Geometry: see drawing. Coordinates: mm, zero at the bounding-box minimum. A direction names the side the tool comes from. Round coordinates to 2 decimals unless told otherwise and drop trailing zeros. Write each loop counter-clockwise with the first axis right and the second up, starting at its lowest first coordinate (ties: lowest second). Pieces come first, ordered by that corner, then holes. Notation, with made-up numbers: M 12.5,-28 L 40.5,-28 A22 ccw 40.5,3 Z; hole C 5.5,31 d5. An arc over 180 degrees is marked long. Use one line per item in the form item = value. Start each with the question number.
Item 1: Reachability of the marked faces 4, 5 and 6 from +Z, -Z, +X, -X, +Y, -Y: full face, straight path, thin tool, end or side. Return the list, or none.
Item 2: Section query B-B (y = 10). Return loops of the section in (x, z), and give its area (3 significant figures).
Item 3: Pin query (flat end, axial travel): pin 1 Ø7 at (x, y) = (10, 10) entering from +Z; pin 2 Ø4 at (x, z) = (3.5, 8) entering from -Y. Return the tip coordinate at first contact, or that it passes through.
Item 4: Pull-direction query (X, two-part tool) for the marked faces 1, 2 and 3; classes: pulls with the +X half, pulls with the -X half, needs draft (parallel to the pull), parting line crosses it, or undercut.
Item 5: Section query A-A (x = 10). Return loops of the section in (y, z).
Item 6: Section query C-C (z = 7.5). Return loops of the section in (x, y), and give its area (3 significant figures).
Item 7: Ray query, probe 1 along Y at (x, z) = (10, 2.25); probe 2 along X at (y, z) = (62, 9.25); probe 3 along Y at (x, z) = (10.5, 2.25). Return the intervals inside material, ascending.
Item 8: Section query D-D (y = 36). Return loops of the section in (x, z).
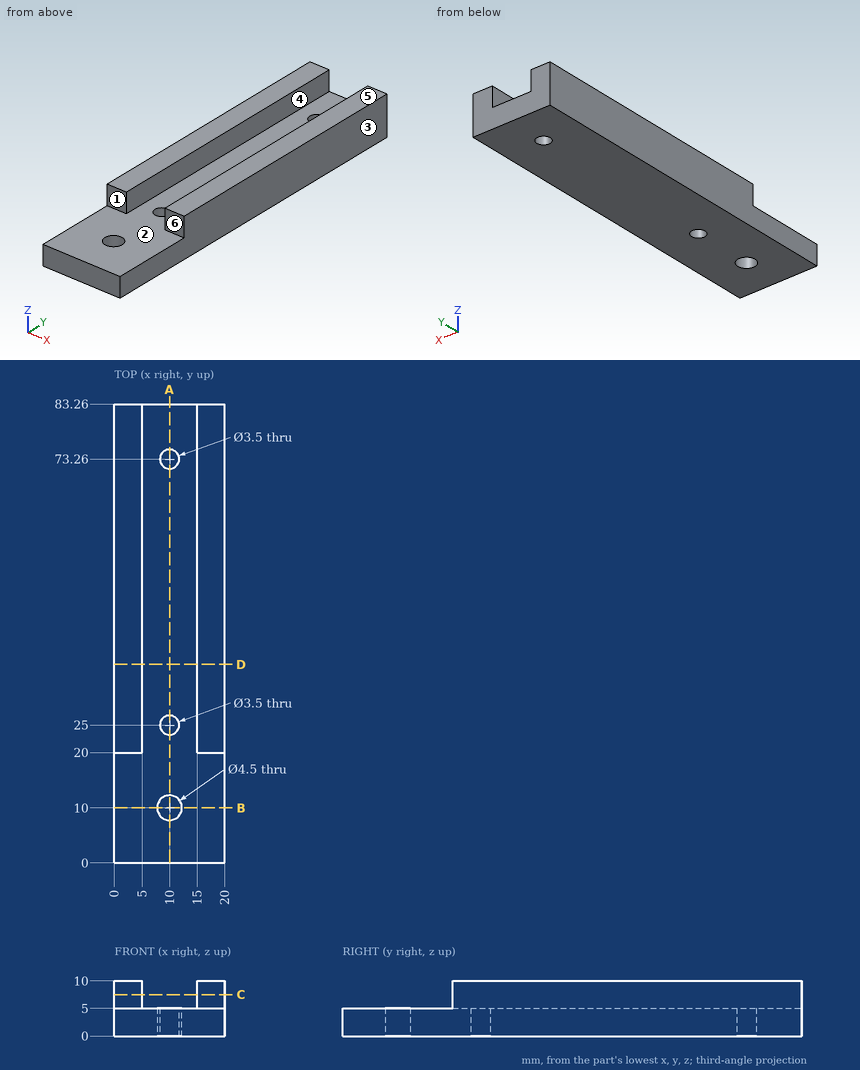
Working result:
q1.face_4 = +Z, +Y, -Y
q1.face_5 = +Z, +X, -X, +Y, -Y
q1.face_6 = +Z, +X, -X, -Y
q2.outline = M 0,0 L 7.75,0 L 7.75,5 L 0,5 Z; M 12.25,0 L 20,0 L 20,5 L 12.25,5 Z
q2.area = 77.5 mm²
q3.pin_1 = 5
q3.pin_2 = 20
q4.face_1 = needs draft
q4.face_2 = undercut
q4.face_3 = pulls with the +X half
q5.outline = M 0,0 L 7.75,0 L 7.75,5 L 0,5 Z; M 12.25,0 L 23.25,0 L 23.25,5 L 12.25,5 Z; M 26.75,0 L 71.51,0 L 71.51,5 L 26.75,5 Z; M 75.01,0 L 83.26,0 L 83.26,5 L 75.01,5 Z
q6.outline = M 0,20 L 5,20 L 5,83.26 L 0,83.26 Z; M 15,20 L 20,20 L 20,83.26 L 15,83.26 Z
q6.area = 633 mm²
q7.probe_1 = 0 to 7.75, 12.25 to 23.25, 26.75 to 71.51, 75.01 to 83.26
q7.probe_2 = 0 to 5, 15 to 20
q7.probe_3 = 0 to 7.81, 12.19 to 23.32, 26.68 to 71.58, 74.94 to 83.26
q8.outline = M 0,0 L 20,0 L 20,10 L 15,10 L 15,5 L 5,5 L 5,10 L 0,10 Z
